CAD build for the part. Positions are in the model's coordinates, mm. A direction names the side the tool comes from. Round coordinates to 2 decimals unless told otherwise and drop trailing zeros. Order: outer loops, then holes, each group sorted by start corner. A loop starts at its lowest first (then second) coordinate and runs counter-clockwise, first axis right, second up. Notation, with made-up numbers: M 76,66.5 L 130,66.5 A16 cw 130,72.5 Z; hole C 47,-7 d6. An arc over 180 degrees is marked long. Answer as CSV lines item,"result". Start each with the question number.
```python
from build123d import *

# Parameters (mm, degrees)
F1_DEPTH = 64.516
F2_T     = -2.54


with BuildPart() as f1:
    # F0 (on Top) → F1 (new body)
    with BuildSketch(Plane.XY):
        Polygon((8.434549, 40.320739), (-35.881834, 24.495647), (-66.348401, -11.367476), (-74.801661, -57.659135), (-58.976569, -101.975517), (-23.113446, -132.442084), (23.178213, -140.895344), (67.494595, -125.070252), (97.961162, -89.207129), (106.414422, -42.915471), (90.58933, 1.400912), (54.726207, 31.867479), align=None)
    extrude(amount=F1_DEPTH)

    # F2
    f2_openings = [f1.faces().sort_by_distance(p)[0] for p in [
        (15.806381, -50.287303, 64.516),
    ]]
    offset(amount=F2_T, openings=f2_openings)


solid = f1.part
```
Q1. Band-saw the part on B-B, the plane x = 45. Write the cut outline in (y, z).
Q2. Band-saw the part on A-A, the plane z = 43. Write the cut outline in (x, y), then the cut area to 3 significant figures.
Q3. Drop flat-ended pins along their axis: P1, Ø5, axis at x = 62, z = 52.5, coming from the +Y side; P2, Ø4, axis at x = -0.5, z = 52, coming from the +Y side; P3, Ø6, axis at y = -75.5, z = 11, coming from the -X side. Give the stop position or say it passes through.
Q4. Tool access for faces 1 (the flat face through (-12.568, 30.124, 33.094)), 2 (the flat face through (-0.29, -136.61, 31.81)): list every direction of +Z, -Z, +X, -X, +Y, -Y with a clear straight run to the whole face (end or side of a thin tool).
Q5. Probe line 1 along Z through (x, y) = (-30, 16); line 2 along X through (y, z) = (-83.5, 53); line 3 along X through (y, z) = (-110, 55). List the from-to ranges inside material, lowest first. Write a range as from..to.
Q6. Mould opens along Y. For faces 3 (the flat face through (-48.972, 5.163, 33.094)), 4 (the flat face through (15, -49, 2.54)), 5 (the flat face through (-13.41, 32.52, 31.81)), 6 (the flat face through (15, -49, 0)) say: +Y half, -Y half, draft (parallel to the pull), parting line (faces both ways), or undercut.
Q7. Band-saw the part on C-C, the plane y = 5. Write the cut outline in (x, z).
Answer:
1,outline,"M -133.1,0 L 33.64,0 L 33.64,64.52 L 31.06,64.52 L 31.06,2.54 L -130.41,2.54 L -130.41,64.52 L -133.1,64.52 Z"
2,outline,"M -74.8,-57.66 L -58.98,-101.98 L -23.11,-132.44 L 23.18,-140.9 L 67.49,-125.07 L 97.96,-89.21 L 106.41,-42.92 L 90.59,1.4 L 54.73,31.87 L 8.43,40.32 L -35.88,24.5 L -66.35,-11.37 Z; hole M -72.18,-57.45 L -56.81,-100.48 L -21.99,-130.07 L 22.96,-138.27 L 66,-122.91 L 95.58,-88.08 L 103.79,-43.13 L 88.43,-0.09 L 53.6,29.49 L 8.65,37.7 L -34.39,22.33 L -63.97,-12.49 Z"
2,area,"1,410 mm^2"
3,P1,"stops at y = 27.81"
3,P2,"stops at y = 37.84"
3,P3,"stops at x = -69.5"
4,face 1,"+Z"
4,face 2,"+Z, -Z, -X, -Y"
5,line 1,"z = 0..2.54"
5,line 2,"x = -65.57..-62.88, 96.42..99"
5,line 3,"x = -49.53..-45.61, 76.96..80.3"
6,face 3,"undercut"
6,face 4,"undercut"
6,face 5,"+Y half"
6,face 6,"draft"
7,outline,"M -52.44,0 L 86.35,0 L 86.35,64.52 L 82.43,64.52 L 82.43,2.54 L -49.11,2.54 L -49.11,64.52 L -52.44,64.52 Z"
